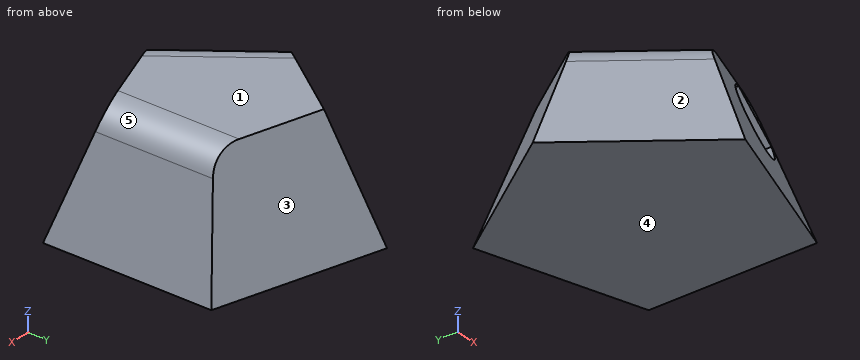
from build123d import *

# Parameters (mm, degrees)
F1_DEPTH = 7
F1_TAPER = 20
F2_R     = 2
F6_DEPTH = 5.3744027906


with BuildPart() as f1:
    # F0 (on Top) → F1 (new body)
    with BuildSketch(Plane.XY):
        Polygon((-2.466497474, -8.1410730242), (6.9804309133, -4.861508412), (6.7806410345, 5.136495589), (-2.7897642884, 8.0360372691), (-8.5048101854, -0.1699514219), align=None)
    extrude(amount=F1_DEPTH, taper=F1_TAPER)

    # F2
    f2_edges = [f1.edges().sort_by_distance(p)[0] for p in [
        (4.333253, 0.086591, 7),
        (-3.454778, -2.617076, 7),
    ]]
    fillet(f2_edges, radius=F2_R)

    # F5 (on face) → F6 (cut, through all)
    with BuildSketch(Plane(origin=(0, 0, 0), x_dir=(0.9998004001, 0.0199789879, 0), z_dir=(0.0199789879, -0.9998004001, 0))):
        with BuildLine():
            Line((4.9218312378, 4.7824094277), (2.4123963387, 6.9308649574))
            ThreePointArc((2.4123963387, 6.9308649574), (1.6329889121, 3.4807425637), (4.9218312378, 4.7824094277))
        make_face()
    extrude(amount=F6_DEPTH, mode=Mode.SUBTRACT)


solid = f1.part
The listing builds one solid part. Answer for the finished solid, in the listing's coordinates (mm). Face numbers are marked on the shaded views. A direction names the side the tool comes from. Coordinates: 2 decimals unless noted, no trailing zeros. Loops run counter-clockwise (first coordinate to the right, second up) from the corner with the lowest first, then second, coordinate; pieces in that order, holes last.
1) A tool of negligible diameter and unlimited length cuts with its end or side. For the marked faces 4 and 5, from which of +Z, -Z, +X, -X, +Y, -Y can it reach the whole face along a straight path? Write none if from no direction.
2) Find section A-A on z = 4. Write down the section's boundary in (x, y), then the cut area to 3 significant figures.
3) Determine the mould class of the marked faces 1, 2 and 3 for opening direction X: pulls with the +X half, pulls with the -X half, needs draft (parallel to the pull), parting line crosses it, or undercut.
4) Find section B-B on y = 4.25. Write down the section's boundary in (x, z), then the cut area to 3 significant figures.
5) Find section C-C on z = 1.5. Write down the section's boundary in (x, y), then the cut area to 3 significant figures.
6) Find section D-D on y = -6.75. Write down the section's boundary in (x, z), then the cut area to 3 significant figures.
7) Flat-ended cylindrical pins translate along their axes: pin 1 Ø2 at (y, z) = (2, 1) entering from -X; pin 2 Ø2 at (x, z) = (4, 1) entering from +Y; pin 3 Ø3 at (x, z) = (-5.5, 2.5) entering from +Y. Find the tip coordinate at first contact, or state that the pin passes through.
8) Find the intervals of material crossed by L1, parallel to X at y = -2.25, z = 3.5; L2, parallel to Y at x = -5.25, z = 4.5; L3, parallel to X at y = -3, z = 6.5, in increasing order.
Values:
1. face 4: -Z, +X, -X, +Y, -Y
1. face 5: +Z, +X, +Y
2. outline: (-6.71, -0.13) - (-1.94, -6.42) - (1.31, -5.29) - (1.2, 0.02) - (4.66, 0.09) - (4.75, -4.1) - (5.5, -3.83) - (5.35, 4.05) - (-2.2, 6.34) - close
2. area: 90.5 mm2
3. face 1: needs draft
3. face 2: pulls with the -X half
3. face 3: pulls with the +X half
4. outline: (-5.43, 0) - (6.8, 0) - (5.61, 3.26) - (0.92, 7) - (-2.32, 7) - close
4. area: 59.6 mm2
5. outline: (-7.83, -0.16) - (-2.27, -7.5) - (6.43, -4.48) - (6.24, 4.73) - (-2.57, 7.4) - close
5. area: 146 mm2
6. outline: (-3.52, 0) - (1.54, 0) - (-2.05, 3.23) - close
6. area: 8.18 mm2
7. pin 1: stops at x = -7.38
7. pin 2: stops at y = 6.08
7. pin 3: stops at y = 4.91
8. L1: x = -5.33 to 1.66, 4.3 to 5.65
8. L2: y = -1.75 to 1.64
8. L3: x = -3.07 to 1.67, 2.98 to 4.32
